Answer from the drawing. Dimensions are ordinates in mm from the lowest x, y and z of the part. Round coordinates to 2 decimals unless told otherwise and drop trailing zeros. Write each loop counter-clockwise with the first axis right and the second up, starting at its lowest first coordinate (ties: lowest second). Pieces come first, ordered by that corner, then holes. Notation, with made-up numbers: M -18,-18.5 L 30,-18.5 A8 cw 30,-12.5 Z; hole C -20,28 d8. An arc over 180 degrees is marked long. One line per item, written item: value. Start each with the question number.
(1) Consider probe 1 along Y at (x, z) = (5, 1.35); probe 2 along X at (y, z) = (13.25, 3.5); probe 3 along X at (y, z) = (11.25, 1.4). Determine where each line is inside the solid, lowest interval first.
(2) Section A-A (y = 12.5) is taken. Determine the outline of the cut face in (x, z), plus the area to 3 significant figures.
(3) Section B-B (x = 105) is taken. Determine the outline of the cut face in (y, z).
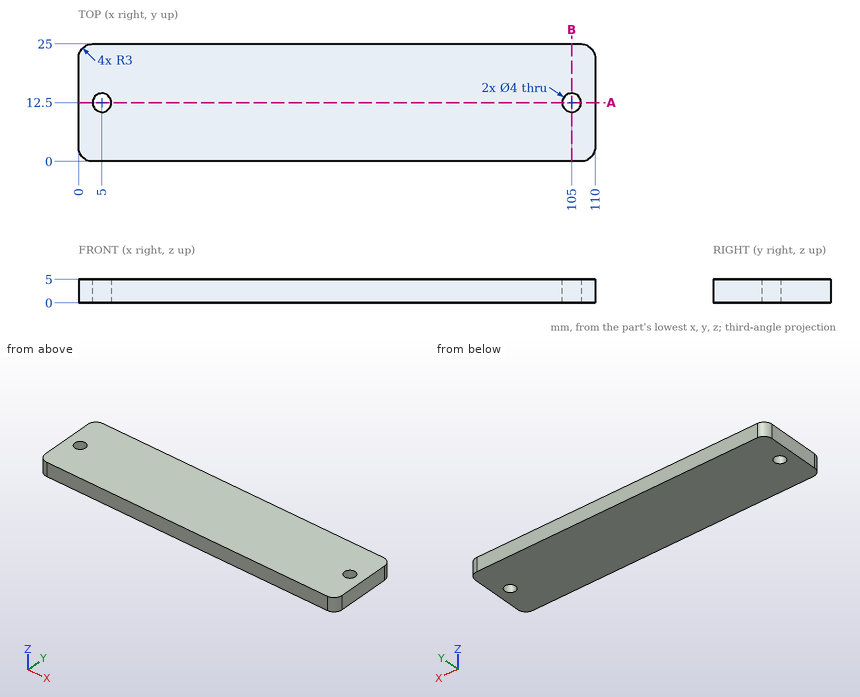
Recorded:
1. probe 1: y = 0 to 10.5, 14.5 to 25
1. probe 2: x = 0 to 3.15, 6.85 to 103.15, 106.85 to 110
1. probe 3: x = 0 to 3.44, 6.56 to 103.44, 106.56 to 110
2. outline: M 0,0 L 3,0 L 3,5 L 0,5 Z; M 7,0 L 103,0 L 103,5 L 7,5 Z; M 107,0 L 110,0 L 110,5 L 107,5 Z
2. area: 510 mm2
3. outline: M 0,0 L 10.5,0 L 10.5,5 L 0,5 Z; M 14.5,0 L 25,0 L 25,5 L 14.5,5 Z
